from build123d import *

# Parameters (mm, degrees)
SKETCH_2_W          = 181
SKETCH_2_H          = 58.5
SKETCH_2_W_2        = 177
SKETCH_2_H_2        = 54.5
EXTRUDE_1_DEPTH     = 30
SKETCH_3_W          = 14.8
SKETCH_3_H          = 58.5
EXTRUDE_2_DEPTH     = 9.9
SKETCH_5_W          = 12.8
SKETCH_5_H          = 54.5
CUT_EXTRUDE_1_DEPTH = 9.9
CUT_EXTRUDE_2_DEPTH = 1000
SKETCH_7_W          = 15
SKETCH_7_H          = 58.5
EXTRUDE_3_DEPTH     = 2


with BuildPart() as part:
    # Эскиз2 → Бобышка-Вытянуть1 (new body)
    with BuildSketch(Plane(origin=(0, 0, 0), x_dir=(1, 0, 0), z_dir=(0, 1, 0))):
        Rectangle(SKETCH_2_W, SKETCH_2_H)
        Rectangle(SKETCH_2_W_2, SKETCH_2_H_2, mode=Mode.SUBTRACT)
    extrude(amount=EXTRUDE_1_DEPTH)

    # Эскиз3 → Бобышка-Вытянуть2 (add)
    with BuildSketch(Plane.XZ):
        with Locations((83.1, 0)):
            Rectangle(SKETCH_3_W, SKETCH_3_H)
    extrude(amount=EXTRUDE_2_DEPTH)

    # Эскиз5 → Вырез-Вытянуть1 (cut)
    with BuildSketch(Plane(origin=(0, 0, 0), x_dir=(1, 0, 0), z_dir=(0, 1, 0))):
        with Locations((82.1, 0)):
            Rectangle(SKETCH_5_W, SKETCH_5_H)
    extrude(amount=-CUT_EXTRUDE_1_DEPTH, mode=Mode.SUBTRACT)

    # Эскиз6 → Вырез-Вытянуть2 (cut)
    with BuildSketch(Plane(origin=(0, 0, -29.25), x_dir=(-1, 0, 0), z_dir=(0, 0, -1))):
        Polygon((-90.5, -9.9), (-75.7, 0), (-75.7, -9.9), align=None)
    extrude(amount=-CUT_EXTRUDE_2_DEPTH, mode=Mode.SUBTRACT)

    # Эскиз7 → Бобышка-Вытянуть3 (add)
    with BuildSketch(Plane(origin=(0, 30, 0), x_dir=(1, 0, 0), z_dir=(0, 1, 0))):
        with Locations((-83, 0)):
            Rectangle(SKETCH_7_W, SKETCH_7_H)
        with Locations((51.997710559, 0)):
            Rectangle(SKETCH_7_W, SKETCH_7_H)
    extrude(amount=-EXTRUDE_3_DEPTH)


solid = part.part
Design review of the part built by this model. Coordinates are the model's own, in mm. A direction names the side the tool comes from. Coordinates: 2 decimals unless noted, no trailing zeros. Order: outer loops, then holes, each group sorted by start corner. A loop starts at its lowest first (then second) coordinate and runs counter-clockwise, first axis right, second up. Notation, with made-up numbers: (-2, 74.25) -> (42, 74.25) arc R27 ccw to (42, 94.25) -> close; hole circle Ø10 at (67, 48.25). An arc over 180 degrees is marked (long way). One line per item, written item: value.
1) Clearance check with flat-ended pins moving along their axes: P1, Ø8, axis at y = -4.5, z = 14, coming from the -X side; P2, Ø6.5, axis at x = -85, z = 6.5, coming from the -Y side. State where each tip first meets the part, or that it passes through.
Output values:
P1: stops at x = 88.5
P2: stops at y = 28
2) Draft analysis for pull direction Z (two halves, no side actions). For faces 1 (the face through (-90.5, 15, 0)), 2 (the face through (-1, 15, 29.25)), 3 (the face through (-82, 28, 0)), state which applies: +Z half, -Z half, draft (parallel to the pull), parting line (faces both ways), or undercut.
Output values:
face 1: draft
face 2: +Z half
face 3: undercut
3) To check wall thickness, follow probe 1 along X at (y, z) = (2.5, 12); probe 2 along Z at (x, y) = (80.5, 15); probe 3 along X at (y, z) = (-3.5, -17). State the ranges of each line that lie inside material, in increasing order. Write a range as [from, to].
Output values:
probe 1: x = [-90.5, -88.5], [88.5, 90.5]
probe 2: z = [-29.25, -27.25], [27.25, 29.25]
probe 3: x = [88.5, 90.5]
4) We need section C-C, the plane z = -2.5. Give the boundary of the cut face in (x, y), then the cut area to 3 significant figures.
Output values:
outline: (-90.5, 0) -> (-88.5, 0) -> (-88.5, 28) -> (-75.5, 28) -> (-75.5, 30) -> (-90.5, 30) -> close; (44.5, 28) -> (59.5, 28) -> (59.5, 30) -> (44.5, 30) -> close; (88.5, -8.56) -> (90.5, -9.9) -> (90.5, 30) -> (88.5, 30) -> close
area: 194 mm2
5) We need section D-D, the plane x = 48. Give the boundary of the cut face in (y, z).
Output values:
outline: (0, -29.25) -> (30, -29.25) -> (30, 29.25) -> (0, 29.25) -> (0, 27.25) -> (28, 27.25) -> (28, -27.25) -> (0, -27.25) -> close
6) Machinability: for faces 4 (the face through (-88.5, 14, 0)), 5 (the face through (-8, 0, -28)), 6 (the face through (88.5, 11, 0)), which of the approach directions +Z, -Z, +X, -X, +Y, -Y give a long, thin tool a straight path to every point of the face, cutting with its end or side? Answer none if there is none.
Output values:
face 4: -Y
face 5: +Z, -Z, -X, -Y
face 6: +Y, -Y
7) We need section B-B, the plane y = 12.5. Give the boundary of the cut face in (x, z).
Output values:
outline: (-90.5, -29.25) -> (90.5, -29.25) -> (90.5, 29.25) -> (-90.5, 29.25) -> close; hole (-88.5, -27.25) -> (88.5, -27.25) -> (88.5, 27.25) -> (-88.5, 27.25) -> close
8) We need section A-A, the plane x = -14.5. Give the boundary of the cut face in (y, z), then the cut area to 3 significant figures.
Output values:
outline: (0, -29.25) -> (30, -29.25) -> (30, -27.25) -> (0, -27.25) -> close; (0, 27.25) -> (30, 27.25) -> (30, 29.25) -> (0, 29.25) -> close
area: 120 mm2
